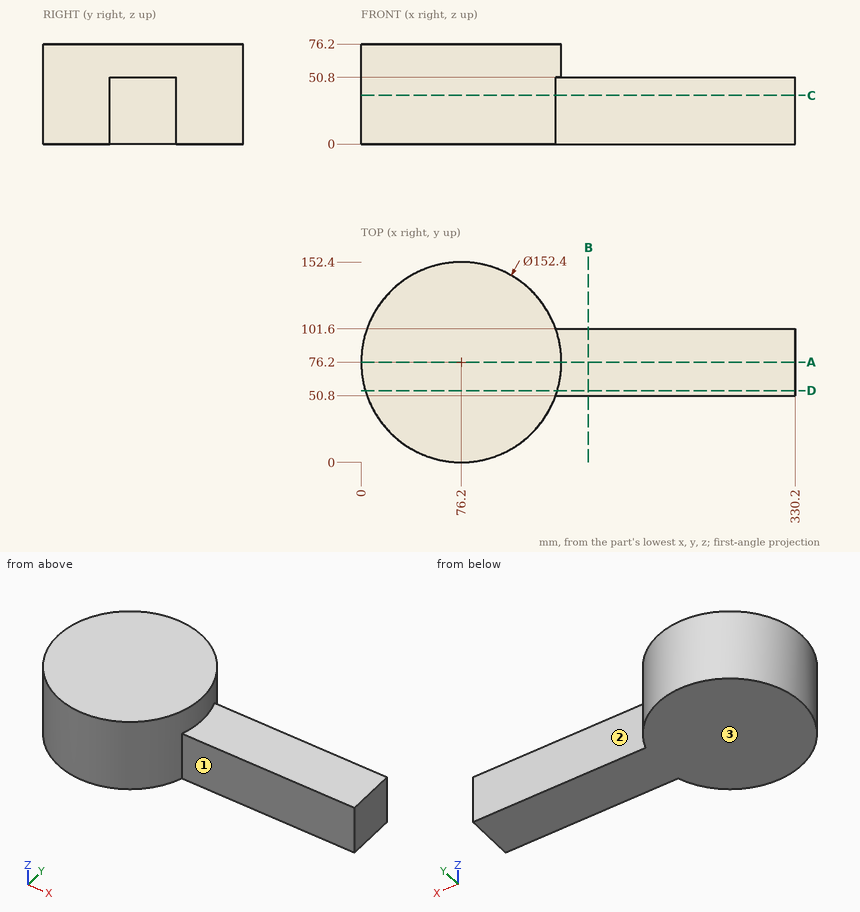
The figure shows three views and two pictorial views of one solid part (mm, origin at its lowest corner). Answer the questions. A direction names the side the tool comes from. Give positions to 0.01 mm unless a question says otherwise; leave off trailing zeros. Loops run counter-clockwise (first coordinate to the right, second up) from the corner with the lowest first, then second, coordinate; pieces in that order, holes last. Notation, with made-up numbers: (29.5, 18.25) -> (55.5, 18.25) arc R11 ccw to (55.5, 34.25) -> close; hole circle Ø2 at (77.5, -24.75). An arc over 180 degrees is marked (long way). Use CSV: the item, a comma, the result in double quotes.
1. The part is cut by section C-C (z = 37). Write down the section's boundary in (x, y), then the cut area to 3 significant figures.
Found:
outline,"(148.04, 50.8) -> (330.2, 50.8) -> (330.2, 101.6) -> (148.04, 101.6) arc R76.2 ccw (long way) to start"
area,"27,300 mm^2"
2. The part is cut by section B-B (x = 173). Write down the section's boundary in (y, z), then the cut area to 3 significant figures.
Found:
outline,"(50.8, 0) -> (101.6, 0) -> (101.6, 50.8) -> (50.8, 50.8) -> close"
area,"2,580 mm^2"
3. The part is cut by section A-A (y = 76.2). Write down the section's boundary in (x, z).
Found:
outline,"(0, 0) -> (330.2, 0) -> (330.2, 50.8) -> (152.4, 50.8) -> (152.4, 76.2) -> (0, 76.2) -> close"
4. A tool of negligible diameter and unlimited length cuts with its end or side. For the marked faces 1, 2 and 3, from which of +Z, -Z, +X, -X, +Y, -Y can it reach the whole face along a straight path? Write none if from no direction.
Found:
face 1,"+Z, -Z, +X, -Y"
face 2,"+Z, -Z, +X, +Y"
face 3,"-Z, +X, -X, +Y, -Y"
5. Straight lines are drawn through the part: line 1 (Z direction, x = 190, y = 57); line 2 (Y direction, x = 215.5, z = 9.5); line 3 (X direction, y = 35, z = 39.5). For each, find the intervals that lie inside material, in ascending order.
Found:
line 1,"0 to 50.8"
line 2,"50.8 to 101.6"
line 3,"12.1 to 140.3"
6. The part is cut by section D-D (y = 54.5). Write down the section's boundary in (x, z), then the cut area to 3 significant figures.
Found:
outline,"(3.16, 0) -> (330.2, 0) -> (330.2, 50.8) -> (149.24, 50.8) -> (149.24, 76.2) -> (3.16, 76.2) -> close"
area,"20,300 mm^2"
7. Flat-ended cylindrical pins translate along their axes: pin 1 Ø8 at (x, y) = (200, 43) entering from -Z; pin 2 Ø3 at (y, z) = (49, 12.5) entering from +X; pin 3 Ø5 at (y, z) = (41, 52) entering from +X; pin 4 Ø12 at (x, z) = (82.5, 15) entering from +Y. Find the tip coordinate at first contact, or state that the pin passes through.
Found:
pin 1,"through"
pin 2,"x = 147.94"
pin 3,"x = 145.03"
pin 4,"y = 152.4"
